Part model, mm, in its own coordinate system. A direction names the side the tool comes from. Coordinates: 2 decimals unless noted, no trailing zeros. Write item = value, one per line.
from build123d import *

# Parameters (mm, degrees)
F0_W     = 48
F0_H     = 27.8
F1_DEPTH = 2
F2_W     = 48
F2_H     = 2
F3_DEPTH = 15.4
F4_W     = 2
F4_H     = 10
F4_H_2   = 2
F5_DEPTH = 25.8
F7_DEPTH = 3
F8_W     = 8
F8_H     = 4.8617787947
F9_DEPTH = 2
F10_R    = 0.99999


# Not quite as in the source:
# - a fillet or chamfer is up to 0.001 mm smaller than in the source, because OpenCascade refuses the exact size


with BuildPart() as f1:
    # F0 (on Front) → F1 (new body)
    with BuildSketch(Plane.XZ):
        with Locations((24, 13.9)):
            Rectangle(F0_W, F0_H)
    extrude(amount=F1_DEPTH)

    # F2 (on face) → F3 (join)
    with BuildSketch(Plane.XZ.offset(2)):
        with Locations((24, 26.8)):
            Rectangle(F2_W, F2_H)
    extrude(amount=F3_DEPTH)

    # F4 (on face) → F5 (join)
    with BuildSketch(Plane(origin=(0, 0, 25.8), x_dir=(1, 0, 0), z_dir=(0, 0, -1))):
        with Locations((47, 7)):
            Rectangle(F4_W, F4_H)
        with Locations((1, 3)):
            Rectangle(F4_W, F4_H_2)
    extrude(amount=F5_DEPTH)

    # F6 (on face) → F7 (join)
    with BuildSketch(Plane(origin=(0, 0, 25.8), x_dir=(1, 0, 0), z_dir=(0, 0, -1))):
        Polygon((46, 15.4), (46, 12), (48, 12), (48, 17.4), (46, 17.4), (2, 17.4), (0, 17.4), (0, 4), (2, 4), (2, 15.4), align=None)
    extrude(amount=F7_DEPTH)

    # F8 (on face) → F9 (cut)
    with BuildSketch(Plane.YZ.offset(48)):
        with Locations((-6, 2.4308893974)):
            Rectangle(F8_W, F8_H)
    extrude(amount=-F9_DEPTH, mode=Mode.SUBTRACT)

    # F10 (radius 1 in the source; OpenCascade refuses exactly that, so slightly less here)
    f10_edges = [f1.edges().sort_by_distance(p)[0] for p in [
        (48, -8.7, 27.8),
        (24, -17.4, 27.8),
        (0, -8.7, 27.8),
        (24, 0, 27.8),
        (48, 0, 13.9),
        (48, -17.4, 25.3),
        (48, -14.7, 22.8),
        (48, -12, 11.4),
        (48, -11, 0),
        (48, -10, 2.430889),
        (48, -6, 4.861779),
        (48, -2, 2.430889),
        (48, -1, 0),
        (0, 0, 13.9),
        (24, 0, 0),
        (0, -17.4, 25.3),
        (24, -17.4, 22.8),
        (0, -10.7, 22.8),
        (0, -4, 11.4),
        (0, -2, 0),
        (47, -2, 4.861779),
        (47, -10, 4.861779),
        (46, -12, 11.4),
        (2, -4, 11.4),
        (2, -9.7, 22.8),
        (46, -13.7, 22.8),
        (24, -15.4, 22.8),
        (1, -4, 0),
        (25, -2, 0),
        (47, -10, 0),
        (46, -11, 0),
        (2, -3, 0),
        (47, -12, 0),
    ]]
    fillet(f10_edges, radius=F10_R)


solid = f1.part
Q1. Mould opens along X. For faces 1 (the face through (46.285, -13.662, 23.101)), 2 (the face through (47.715, -8.592, 27.499)), 3 (the face through (24, 0, 14)) say: released by +X, released by -X, zero draft, split by the parting line, or undercut.
Model answer:
face_1 = undercut
face_2 = released by +X
face_3 = zero draft
Q2. Pin check, flat tips, straight feed: pin 1 (10 mm diameter, centred on x = 39, y = -2, fed in from -Z); pin 2 (12.5 mm diameter, centred on x = 16, z = 9, fed in from -Y); pin 3 (4 mm diameter, centred on x = 14, y = -7.5, fed in from -Z); pin 4 (4 mm diameter, centred on y = -6.5, z = 13.5, fed in from -X). Stop position of each tip, or through.
Model answer:
pin_1 = 0
pin_2 = -2
pin_3 = 25.8
pin_4 = 46
Q3. Probe line 1 (X direction, y = -12.5, z = 24.75); line 2 (Y direction, x = 22, z = 5.25); line 3 (X direction, y = -8.5, z = 22.5). List the from-to ranges inside material, lowest first. Write a range as from..to.
Model answer:
line_1 = 0..2, 46..48
line_2 = -2..0
line_3 = 46..48
Q4. Which spindle directions (+Z, -Z, +X, -X, +Y, -Y) get a long thin tool onto all of the face, cutting with end or side? Do faces 4 (the face through (0.285, -3.699, 12.24)), 5 (the face through (1.699, -9.794, 23.085)), 6 (the face through (47.699, -10.285, 2.451)), 7 (the face through (47.715, -0.301, 14.081)). Say none if no direction does.
Model answer:
face_4 = -Z, -X, -Y
face_5 = -Z
face_6 = -Z, +X
face_7 = +Z, -Z, +X, +Y
